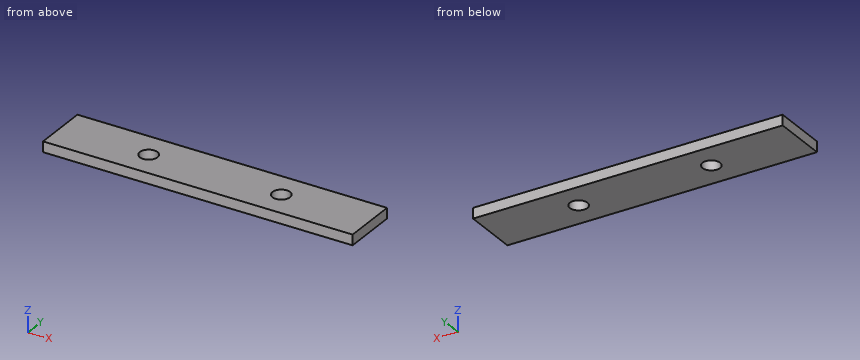
```python
from build123d import *

# Parameters (mm, degrees)
SKETCH1_W           = 88.9
SKETCH1_H           = 15.875
BOSS_EXTRUDE1_DEPTH = 1.4986
SKETCH2_R           = 2.54
CUT_EXTRUDE1_DEPTH  = 3.9972


with BuildPart() as part:
    # Sketch1 → Boss-Extrude1 (new body, symmetric)
    with BuildSketch(Plane.XY):
        Rectangle(SKETCH1_W, SKETCH1_H)
    extrude(amount=BOSS_EXTRUDE1_DEPTH, both=True)

    # Sketch2 → Cut-Extrude1 (cut, through all)
    with BuildSketch(Plane(origin=(0, 0, -1.4986), x_dir=(-1, 0, 0), z_dir=(0, 0, -1))):
        with Locations((-19.05, 0)):
            Circle(SKETCH2_R)
        with Locations((19.05, 0)):
            Circle(SKETCH2_R)
    extrude(amount=-CUT_EXTRUDE1_DEPTH, mode=Mode.SUBTRACT)


solid = part.part
```
For this review, take the finished solid that the model builds, in its own axes (mm). Give positions to 0.01 mm unless a question says otherwise; leave off trailing zeros. Loops run counter-clockwise (first coordinate to the right, second up) from the corner with the lowest first, then second, coordinate; pieces in that order, holes last. Notation, with made-up numbers: M -1,75 L 54,75 A19 ccw 54,99 Z; hole C 45.5,29 d2. An arc over 180 degrees is marked long. One line per item, written item: value. Start each with the question number.
Q1. Add section B-B (x = 19.05). Give the boundary of the cut face in (y, z).
Q2. Add section C-C (z = 0.7). Give the boundary of the cut face in (x, y), and give its area (3 significant figures).
Q3. For L1, parallel to X at y = -0.25, z = 1.15; L2, parallel to Y at x = -19.05, z = 0.05; L3, parallel to X at y = -2.25, z = 1.2, list the stretches that pass through material, from the lowest coordinate up.
Q4. Add section A-A (y = 0). Give the boundary of the cut face in (x, z), and give its area (3 significant figures).
Reply:
1. outline: M -7.94,-1.5 L -2.54,-1.5 L -2.54,1.5 L -7.94,1.5 Z; M 2.54,-1.5 L 7.94,-1.5 L 7.94,1.5 L 2.54,1.5 Z
2. outline: M -44.45,-7.94 L 44.45,-7.94 L 44.45,7.94 L -44.45,7.94 Z; hole C -19.05,0 d5.08; hole C 19.05,0 d5.08
2. area: 1,370 mm²
3. L1: -44.45 to -21.58, -16.52 to 16.52, 21.58 to 44.45
3. L2: -7.94 to -2.54, 2.54 to 7.94
3. L3: -44.45 to -20.23, -17.87 to 17.87, 20.23 to 44.45
4. outline: M -44.45,-1.5 L -21.59,-1.5 L -21.59,1.5 L -44.45,1.5 Z; M -16.51,-1.5 L 16.51,-1.5 L 16.51,1.5 L -16.51,1.5 Z; M 21.59,-1.5 L 44.45,-1.5 L 44.45,1.5 L 21.59,1.5 Z
4. area: 236 mm²
